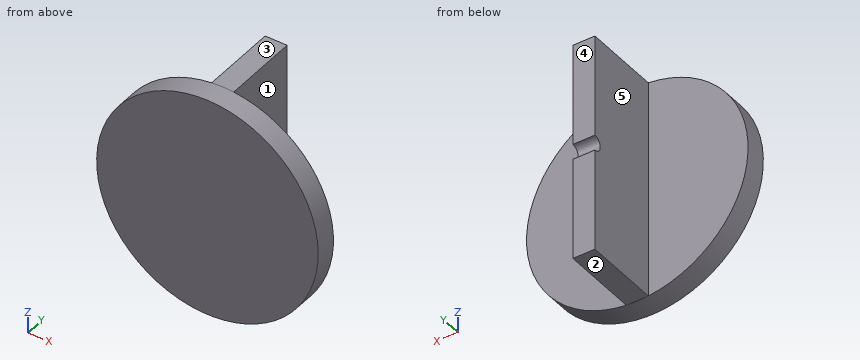
from build123d import *

# Parameters (mm, degrees)
BOSS_EXTRUDE1_DEPTH = 5
SKETCH2_R           = 50.249378106
BOSS_EXTRUDE2_DEPTH = 10


with BuildPart() as part:
    # Sketch1 → Boss-Extrude1 (new, symmetric)
    with BuildSketch(Plane(origin=(0, 0, 0), x_dir=(0, 0, -1), z_dir=(1, 0, 0))):
        with BuildLine():
            Line((-3.5, 17.5), (-50, 17.5))
            Line((-50, 17.5), (-50, -17.5))
            Line((-50, -17.5), (50, -17.5))
            Line((50, -17.5), (50, 17.5))
            Line((50, 17.5), (3.5, 17.5))
            ThreePointArc((3.5, 17.5), (0, 14), (-3.5, 17.5))
        make_face()
    extrude(amount=BOSS_EXTRUDE1_DEPTH, both=True)

    # Sketch2 → Boss-Extrude2 (add)
    with BuildSketch(Plane.XZ.offset(17.5)):
        with Locations(Location((0, 0, 0), (0, 0, 95.710593137))):
            Circle(SKETCH2_R)
    extrude(amount=BOSS_EXTRUDE2_DEPTH)


solid = part.part
Here's how the part is built. I have some questions about the finished solid (model axes, mm). Face numbers are marked on the shaded views. A direction names the side the tool comes from. Coordinates: 2 decimals unless noted, no trailing zeros. Order: outer loops, then holes, each group sorted by start corner. A loop starts at its lowest first (then second) coordinate and runs counter-clockwise, first axis right, second up. Notation, with made-up numbers: (88, 68.25) - (141, 68.25) arc R36 cw to (141, 105.25) - close; hole circle Ø8 at (69.25, 86). An arc over 180 degrees is marked (long way). Use CSV: the item, a comma, the result in double quotes. Start each with the question number.
1. I'm going to push flat-ended pins straight in: pin 1 (12 mm diameter, centred on y = -12, z = -7.5, fed in from -X); pin 2 (8 mm diameter, centred on x = -1, y = 6, fed in from +Z); pin 3 (1.5 mm diameter, centred on y = -12.5, z = 24, fed in from +X). Where does each tip first touch, or does it pass through?
2. Please list where these lines run through material, in increasing order: line 1 (Y direction, x = -22, z = -24.5); line 2 (X direction, y = -15, z = 0); line 3 (Z direction, x = 4.5, y = -7.5). Write a range as from..to.
3. For the marked faces 1, 2, 3, 4 and 5, which set-ups out of +Z, -Z, +X, -X, +Y, -Y let a thin tool reach every point of the face, with its end or its side?
4. Suppose I cut it at C-C on z = -11. List the corners of the cut face in (x, y) for me, then the cut area to 3 significant figures.
5. Suppose I cut it at D-D on x = 7.5. List the corners of the cut face in (y, z) for me.
6. Suppose I cut it at A-A on z = 0. List the corners of the cut face in (x, y) for me, then the cut area to 3 significant figures.
7. Suppose I cut it at B-B on y = -15. List the corners of the cut face in (x, z) for me.
Output:
1,pin 1,"stops at x = -49.99"
1,pin 2,"stops at z = 50"
1,pin 3,"stops at x = 5"
2,line 1,"y = -27.5..-17.5"
2,line 2,"x = -5..5"
2,line 3,"z = -50..50"
3,face 1,"+Z, -Z, +X, +Y"
3,face 2,"-Z, +X, -X, +Y"
3,face 3,"+Z, +X, -X, +Y"
3,face 4,"+Z, -Z, +X, -X, +Y"
3,face 5,"+Z, -Z, -X, +Y"
4,outline,"(-49.03, -27.5) - (49.03, -27.5) - (49.03, -17.5) - (5, -17.5) - (5, 17.5) - (-5, 17.5) - (-5, -17.5) - (-49.03, -17.5) - close"
4,area,"1,330 mm2"
5,outline,"(-27.5, -49.69) - (-17.5, -49.69) - (-17.5, 49.69) - (-27.5, 49.69) - close"
6,outline,"(-50.25, -27.5) - (50.25, -27.5) - (50.25, -17.5) - (5, -17.5) - (5, 14) - (-5, 14) - (-5, -17.5) - (-50.25, -17.5) - close"
6,area,"1,320 mm2"
7,outline,"(-5, -50) - (5, -50) - (5, 50) - (-5, 50) - close"
